Model file for the job. Use its own axes, mm. Face numbers are marked on the shaded views. A direction names the side the tool comes from. Round coordinates to 2 decimals unless told otherwise and drop trailing zeros. Order: outer loops, then holes, each group sorted by start corner. A loop starts at its lowest first (then second) coordinate and runs counter-clockwise, first axis right, second up. Notation, with made-up numbers: (42, -4) - (52, -4) arc R17 cw to (52, 4) - close; hole circle Ø6 at (62.25, -20). An arc over 180 degrees is marked (long way). Write item = value, one per line.
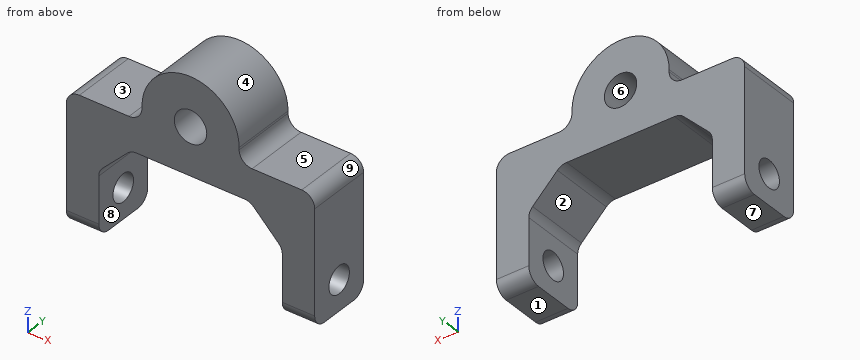
```python
from build123d import *

# Parameters (mm, degrees)
BOSS_EXTRUDE1_DEPTH = 12.7
SKETCH2_R           = 2.667
CUT_EXTRUDE1_DEPTH  = 49.6664
BOSS_EXTRUDE3_DEPTH = 12.7
BOSS_EXTRUDE4_DEPTH = 12.7
CUT_EXTRUDE2_REACH  = 14.7
SKETCH5_R           = 3.175
FILLET1_R           = 2.54
RR_R                = 2.54
FILLET3_R           = 2.54


with BuildPart() as part:
    # Sketch1 → Boss-Extrude1 (new body)
    with BuildSketch(Plane(origin=(0, 0, 0), x_dir=(1, 0, 0), z_dir=(0, 1, 0))):
        Polygon((-6.35, -6.35), (-6.35, 19.05), (0, 19.05), (0, 0), (35.9664, 0), (35.9664, 19.05), (42.3164, 19.05), (42.3164, -6.35), align=None)
    extrude(amount=BOSS_EXTRUDE1_DEPTH)

    # Sketch2 → Cut-Extrude1 (cut, through all)
    with BuildSketch(Plane(origin=(42.3164, 0, 0), x_dir=(0, 0, -1), z_dir=(1, 0, 0))):
        with Locations((13.081, 6.35)):
            Circle(SKETCH2_R)
    extrude(amount=-CUT_EXTRUDE1_DEPTH, mode=Mode.SUBTRACT)

    # Sketch3 → Boss-Extrude3 (add)
    with BuildSketch(Plane(origin=(0, 12.7, 0), x_dir=(1, 0, 0), z_dir=(0, 1, 0))):
        Polygon((0, 0), (6.35, 0), (0, 6.35), align=None)
        Polygon((35.9664, 6.35), (29.6164, 0), (35.9664, 0), align=None)
    extrude(amount=-BOSS_EXTRUDE3_DEPTH)

    # Sketch4 → Boss-Extrude4 (add)
    with BuildSketch(Plane.XZ):
        with BuildLine():
            Line((27.5082, 9.32613509), (27.5082, 6.35))
            Line((27.5082, 6.35), (8.4582, 6.35))
            Line((8.4582, 6.35), (8.4582, 9.32613509))
            ThreePointArc((8.4582, 9.32613509), (17.9832, 18.85113509), (27.5082, 9.32613509))
        make_face()
    extrude(amount=-BOSS_EXTRUDE4_DEPTH)

    # Sketch5 → Cut-Extrude2 (cut, up to next)
    with BuildSketch(Plane.XZ, mode=Mode.PRIVATE) as cut_extrude2_sk1:
        with Locations((17.9832, 9.32613509)):
            Circle(SKETCH5_R)
    cut_extrude2_tool1 = extrude(cut_extrude2_sk1.sketch, amount=-CUT_EXTRUDE2_REACH, mode=Mode.PRIVATE) & part.part
    add(cut_extrude2_tool1.solids().sort_by_distance((17.9832, 0, 9.326135))[0], mode=Mode.SUBTRACT)

    # Fillet1
    fillet1_edges = [part.edges().sort_by_distance(p)[0] for p in [
        (42.3164, 6.35, 6.35),
        (-6.35, 6.35, 6.35),
        (8.4582, 6.35, 6.35),
        (27.5082, 6.35, 6.35),
    ]]
    fillet(fillet1_edges, radius=FILLET1_R)

    # rr
    rr_edges = [part.edges().sort_by_distance(p)[0] for p in [
        (0, 6.35, -6.35),
        (6.35, 6.35, 0),
        (35.9664, 6.35, -6.35),
        (29.6164, 6.35, 0),
    ]]
    fillet(rr_edges, radius=RR_R)

    # Fillet3
    fillet3_edges = [part.edges().sort_by_distance(p)[0] for p in [
        (-3.175, 0, -19.05),
        (39.1414, 12.7, -19.05),
        (-3.175, 12.7, -19.05),
        (39.1414, 0, -19.05),
    ]]
    fillet(fillet3_edges, radius=FILLET3_R)


solid = part.part
```
1) Wall check: line 1 along Z through (x, y) = (-1, 6.5); line 2 along Z through (x, y) = (39.5, 6.25); line 3 along X through (y, z) = (10, -12.5). Give the ranges that are in metal, low to high.
Conclusion:
line_1 = -19.05 to -15.74, -10.42 to 6.35
line_2 = -19.05 to -15.75, -10.42 to 6.35
line_3 = -6.35 to 0, 35.97 to 42.32
2) Mould opens along Z. For the marked faces 6, 7, 8 and 9 say: +Z half, -Z half, draft (parallel to the pull), parting line (faces both ways), or undercut.
Conclusion:
face_6 = undercut
face_7 = -Z half
face_8 = draft
face_9 = +Z half
3) Cut at B-B (y = 6.35). Give the number of separate pieces and of enclosed holes in the cut face, and give its area (3 significant figures).
Conclusion:
separate_pieces = 3
enclosed_holes = 1
area = 692 mm^2
4) 3-axis set-ups, long thin cutter, end or side, ignore diameter. For the marked faces 1, 2, 3, 4 and 5: which of +Z, -Z, +X, -X, +Y, -Y reach the whole face in a straight line?
Conclusion:
face_1 = -Z, +X, -X, +Y, -Y
face_2 = -Z, +Y, -Y
face_3 = +Z, -X, +Y, -Y
face_4 = +Z, +Y, -Y
face_5 = +Z, +X, +Y, -Y
5) Cut at A-A (x = 38.5). Write the cut outline in (y, z), and give its area (3 significant figures).
Conclusion:
outline = (0, -16.51) arc R2.54 ccw to (2.54, -19.05) - (10.16, -19.05) arc R2.54 ccw to (12.7, -16.51) - (12.7, 6.35) - (0, 6.35) - close; hole circle Ø5.33 at (6.35, -13.08)
area = 297 mm^2
6) Cut at D-D (z = -14). Write the cut outline in (x, y), and give its area (3 significant figures).
Conclusion:
outline = (-6.35, 0) - (0, 0) - (0, 3.85) - (-6.35, 3.85) - close; (-6.35, 8.85) - (0, 8.85) - (0, 12.7) - (-6.35, 12.7) - close; (35.97, 0) - (42.32, 0) - (42.32, 3.85) - (35.97, 3.85) - close; (35.97, 8.85) - (42.32, 8.85) - (42.32, 12.7) - (35.97, 12.7) - close
area = 97.7 mm^2
7) Flat gauge pins, fed straight in: pin 1 Ø3 at (x, y) = (0, 8.5) entering from +Z; pin 2 Ø0.5 at (y, z) = (7, 9) entering from +X; pin 3 Ø2 at (y, z) = (6, 12) entering from -X. Where does each tip first touch, or does it go through?
Conclusion:
pin_1 = 6.35
pin_2 = 27.51
pin_3 = 8.61
8) Cut at C-C (z = -4.5). Write the cut outline in (x, y).
Conclusion:
outline = (-6.35, 0) - (1.85, 0) - (1.85, 12.7) - (-6.35, 12.7) - close; (34.12, 0) - (42.32, 0) - (42.32, 12.7) - (34.12, 12.7) - close
